```python
from build123d import *

# Parameters (mm, degrees)
F0_W     = 127.5347471237
F0_H     = 50.8334226906
F1_DEPTH = 50.8
F2_DEPTH = 32.766
F3_W     = 53.2384
F3_H     = 30.988
F4_DEPTH = 33.528
F5_DEPTH = 4.826
F6_DEPTH = 7.366
F7_DEPTH = 8.89
F8_DEPTH = 9.652
F9_DEPTH = 5.334


with BuildPart() as f1:
    # F0 (on Front) → F1 (new body)
    with BuildSketch(Plane.XZ):
        with Locations((63.7673735619, 25.4167113453)):
            Rectangle(F0_W, F0_H)
    extrude(amount=F1_DEPTH)

    # F2 (cut): a face of the model
    f2_faces = [f1.faces().sort_by_distance(p)[0] for p in [
        (63.7673735619, -25.4, 50.8334226906),
    ]]
    extrude(f2_faces, amount=-F2_DEPTH, mode=Mode.SUBTRACT)

    # F3 (on face) → F4 (join)
    with BuildSketch(Plane.XY.offset(18.0674226906)):
        with Locations((65.5213113515, -15.494)):
            Rectangle(F3_W, F3_H)
    extrude(amount=F4_DEPTH)

    # F5 (cut): a face of the model
    f5_faces = [f1.faces().sort_by_distance(p)[0] for p in [
        (127.5347471237, -25.4, 9.0337113453),
    ]]
    extrude(f5_faces, amount=-F5_DEPTH, mode=Mode.SUBTRACT)

    # F6 (add): a face of the model
    f6_faces = [f1.faces().sort_by_distance(p)[0] for p in [
        (0, -25.4, 9.0337113453),
    ]]
    extrude(f6_faces, amount=-F6_DEPTH)

    # F7 (add): a face of the model
    f7_faces = [f1.faces().sort_by_distance(p)[0] for p in [
        (0, -25.4, 9.0337113453),
    ]]
    extrude(f7_faces, amount=-F7_DEPTH)

    # F8 (cut): a face of the model
    f8_faces = [f1.faces().sort_by_distance(p)[0] for p in [
        (0, -25.4, 9.0337113453),
    ]]
    extrude(f8_faces, amount=-F8_DEPTH, mode=Mode.SUBTRACT)

    # F9 (add): a face of the model
    f9_faces = [f1.faces().sort_by_distance(p)[0] for p in [
        (66.1803735619, -50.8, 9.0337113453),
    ]]
    extrude(f9_faces, amount=-F9_DEPTH)


solid = f1.part
```
Build history of the part. All positions in model axes, mm. A direction names the side the tool comes from. Give positions to 0.01 mm unless a question says otherwise; leave off trailing zeros. Loops run counter-clockwise (first coordinate to the right, second up) from the corner with the lowest first, then second, coordinate; pieces in that order, holes last.
Item 1: Which spindle directions (+Z, -Z, +X, -X, +Y, -Y) get a long thin tool onto all of the face, cutting with end or side? Do faces 1 (the face through (92.141, -16, 35)), 2 (the face through (38.902, -16, 35)), 3 (the face through (65, -30.988, 35)), 4 (the face through (122.709, -26, 9)). Say none if no direction does.
Answers follow:
face 1: +Z, +X, +Y, -Y
face 2: +Z, -X, +Y, -Y
face 3: +Z, +X, -X, -Y
face 4: +Z, -Z, +X, +Y, -Y
Item 2: Slice it at D-D, the plane x = 108. List the corners of the cut face in (y, z).
Answers follow:
outline: (-50.8, 0) - (0, 0) - (0, 18.07) - (-50.8, 18.07) - close
Item 3: Drill centre lines: line 1 (Z direction, x = 32, y = -23); line 2 (X direction, y = -13, z = 33.5); line 3 (Y direction, x = 90.5, z = 26.5). Where is each one in solid material? Low to high.
Answers follow:
line 1: z = 0 to 18.07
line 2: x = 38.9 to 92.14
line 3: y = -30.99 to 0
Item 4: Slice it at C-C, the plane z = 47. List the corners of the cut face in (x, y).
Answers follow:
outline: (38.9, -30.99) - (92.14, -30.99) - (92.14, 0) - (38.9, 0) - close
Item 5: Slice it at A-A, the plane y = -22. List the corners of the cut face in (x, z), and give its area (3 significant figures).
Answers follow:
outline: (9.65, 0) - (122.71, 0) - (122.71, 18.07) - (92.14, 18.07) - (92.14, 51.6) - (38.9, 51.6) - (38.9, 18.07) - (9.65, 18.07) - close
area: 3,830 mm2
Item 6: Slice it at B-B, the plane x = 46.5. List the corners of the cut face in (y, z).
Answers follow:
outline: (-50.8, 0) - (0, 0) - (0, 51.6) - (-30.99, 51.6) - (-30.99, 18.07) - (-50.8, 18.07) - close
Item 7: Flat gauge pins, fed straight in: pin 1 (1 mm diameter, centred on x = 32, z = 16, fed in from +Y); pin 2 (15.5 mm diameter, centred on y = -9, z = 28, fed in from -X); pin 3 (1.5 mm diameter, centred on y = -6, z = 37.5, fed in from +X). Where does each tip first touch, or does it go through?
Answers follow:
pin 1: stops at y = 0
pin 2: stops at x = 38.9
pin 3: stops at x = 92.14
